Geometry: final body of the model. Coordinates: model frame, mm. Face numbers are marked on the shaded views. A direction names the side the tool comes from. Round coordinates to 2 decimals unless told otherwise and drop trailing zeros. Write each loop counter-clockwise with the first axis right and the second up, starting at its lowest first coordinate (ties: lowest second). Pieces come first, ordered by that corner, then holes. Notation, with made-up numbers: M -34,-39 L -13,-39 A21 ccw -13,-21 Z; hole C 4.5,83 d10. An arc over 180 degrees is marked long. Use one line per item in the form item = value. Start each with the question number.
Item 1: Reachability of the marked faces 4 and 5 from +Z, -Z, +X, -X, +Y, -Y: full face, straight path, thin tool, end or side. Return the list, or none.
Item 2: Pin query (flat end, axial travel): pin 1 Ø1.4 at (x, z) = (9, 12.5) entering from +Y; pin 2 Ø3.5 at (x, z) = (9, 14.5) entering from -Y; pin 3 Ø6 at (x, y) = (-20, 4) entering from +Z. Return the tip coordinate at first contact, or that it passes through.
Item 3: Section query D-D (z = 16). Return loops of the section in (x, y).
Item 4: Ray query, probe 1 along Y at (x, z) = (-4, 12.25); probe 2 along X at (y, z) = (-6.5, 3); probe 3 along X at (y, z) = (-6.25, 4). Return the intervals inside material, ascending.
Item 5: Section query B-B (z = 2.75). Return loops of the section in (x, y).
Item 6: Pull-direction query (X, two-part tool) for the marked faces 1, 2 and 3; classes: pulls with the +X half, pulls with the -X half, needs draft (parallel to the pull), parting line crosses it, or undercut.
Item 7: Section query C-C (x = -6). Return loops of the section in (y, z), and give its area (3 significant figures).
Item 8: Section query A-A (y = 0). Return loops of the section in (x, z).
from build123d import *

# Parameters (mm, degrees)
F1_DEPTH = 20
F2_DEPTH = 5.8
F3_R     = 2.1592673483
F4_DEPTH = 25


# Not quite as in the source:
# - a feature names something its author has since deleted; it is built from what else it names


with BuildPart() as f1:
    # F0 (on Top) → F1 (new body)
    with BuildSketch(Plane.XY):
        with BuildLine():
            ThreePointArc((7.5199086274, -1.1004427451), (-7.6, 0), (7.5199086274, 1.1004427451))
            Line((7.5199086274, 1.1004427451), (12.0555223817, 1.1004427451))
            Line((12.0555223817, 1.1004427451), (12.0555223817, 5.7252630293))
            Line((12.0555223817, 5.7252630293), (11.1117668822, 5.7252630293))
            ThreePointArc((11.1117668822, 5.7252630293), (6.5070812248, 10.6727641187), (0, 12.5))
            Line((0, 12.5), (-10.78635397, 12.5))
            Line((-10.78635397, 12.5), (-10.78635397, 4.5))
            Line((-10.78635397, 4.5), (-10.78635397, -4.5))
            Line((-10.78635397, -4.5), (-10.78635397, -12.5))
            Line((-10.78635397, -12.5), (0, -12.5))
            ThreePointArc((0, -12.5), (7.0722638762, -10.3069434687), (11.6629478347, -4.4972933866))
            Line((11.6629478347, -4.4972933866), (12.0555223817, -4.4972933866))
            Line((12.0555223817, -4.4972933866), (12.0555223817, -1.1004427451))
            Line((12.0555223817, -1.1004427451), (7.5199086274, -1.1004427451))
        make_face()
    extrude(amount=F1_DEPTH)

    # F0 (on Top) → F2 (join)
    with BuildSketch(Plane.XY):
        Polygon((-10.78635397, 4.5), (-10.78635397, 12.5), (-30.2485086955, 12.5), (-30.2485086955, -4.5), (-30.2485086955, -12.5), (-10.78635397, -12.5), (-10.78635397, -4.5), align=None)
    extrude(amount=F2_DEPTH)

    # F3 (on face) → F4 (cut)
    with BuildSketch(Plane.XY.offset(5.8)):
        with Locations((-20.5174313327, 0)):
            Circle(F3_R)
    extrude(amount=-F4_DEPTH, mode=Mode.SUBTRACT)


solid = f1.part
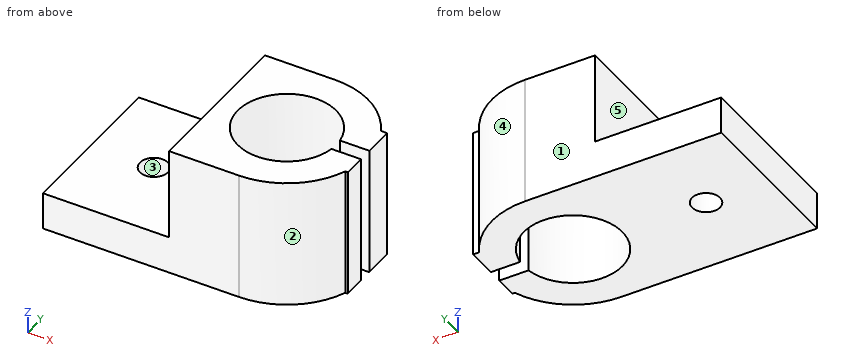
Working result:
q1.face_4 = +Z, -Z, +X, +Y
q1.face_5 = +Z, -X, +Y, -Y
q2.pin_1 = 9.35
q2.pin_2 = -10.18
q2.pin_3 = 5.8
q3.outline = M -10.79,-12.5 L 0,-12.5 A12.5 ccw 11.66,-4.5 L 12.06,-4.5 L 12.06,-1.1 L 7.52,-1.1 A7.6 cw long 7.52,1.1 L 12.06,1.1 L 12.06,5.73 L 11.11,5.73 A12.5 ccw 0,12.5 L -10.79,12.5 Z
q4.probe_1 = -12.5 to -6.46, 6.46 to 12.5
q4.probe_2 = -30.25 to -3.94, 3.94 to 10.68
q4.probe_3 = -30.25 to -4.32, 4.32 to 10.83
q5.outline = M -30.25,-12.5 L 0,-12.5 A12.5 ccw 11.66,-4.5 L 12.06,-4.5 L 12.06,-1.1 L 7.52,-1.1 A7.6 cw long 7.52,1.1 L 12.06,1.1 L 12.06,5.73 L 11.11,5.73 A12.5 ccw 0,12.5 L -30.25,12.5 Z; hole C -20.52,0 d4.32
q6.face_1 = needs draft
q6.face_2 = pulls with the +X half
q6.face_3 = undercut
q7.outline = M -12.5,0 L -4.66,0 L -4.66,20 L -12.5,20 Z; M 4.66,0 L 12.5,0 L 12.5,20 L 4.66,20 Z
q7.area = 313 mm²
q8.outline = M -30.25,0 L -22.68,0 L -22.68,5.8 L -30.25,5.8 Z; M -18.36,0 L -7.6,0 L -7.6,20 L -10.79,20 L -10.79,5.8 L -18.36,5.8 Z
